from build123d import *

# Parameters (mm, degrees)
SKETCH1_R           = 5
SKETCH1_R_2         = 3
BOSS_EXTRUDE2_DEPTH = 0.5
CUT_EXTRUDE5_DEPTH  = 0.2


with BuildPart() as part:
    # Sketch1 → Boss-Extrude2 (new body)
    with BuildSketch(Plane(origin=(0, 0, 0), x_dir=(1, 0, 0), z_dir=(0, 1, 0))):
        Circle(SKETCH1_R)
        Circle(SKETCH1_R_2, mode=Mode.SUBTRACT)
    extrude(amount=BOSS_EXTRUDE2_DEPTH)

    # Sketch4 → Cut-Extrude5 (cut)
    with BuildSketch(Plane(origin=(0, 0, 0), x_dir=(1, 0, 0), z_dir=(0, 1, 0))):
        with BuildLine():
            Line((-1.227705378, 2.901045691), (-4.555523725, 1.283756278))
            ThreePointArc((-4.555523725, 1.283756278), (-4.689175287, 1.32998679), (-4.642944775, 1.463638351))
            Line((-4.642944775, 1.463638351), (-1.315126427, 3.080927764))
            ThreePointArc((-1.315126427, 3.080927764), (-1.181474866, 3.034697252), (-1.227705378, 2.901045691))
        make_face()
        with BuildLine():
            Line((0.388990404, 3.128300785), (-3.301629531, 3.391596243))
            ThreePointArc((-3.301629531, 3.391596243), (-3.394259922, 3.498458821), (-3.287397344, 3.591089212))
            Line((-3.287397344, 3.591089212), (0.403222591, 3.327793755))
            ThreePointArc((0.403222591, 3.327793755), (0.495852982, 3.220931177), (0.388990404, 3.128300785))
        make_face()
        with BuildLine():
            Line((1.902717568, 2.516761579), (-1.161805322, 4.590092101))
            ThreePointArc((-1.161805322, 4.590092101), (-1.188594305, 4.728953005), (-1.049733402, 4.755741987))
            Line((-1.049733402, 4.755741987), (2.014789488, 2.682411465))
            ThreePointArc((2.014789488, 2.682411465), (2.041578471, 2.543550562), (1.902717568, 2.516761579))
        make_face()
        with BuildLine():
            Line((2.907874144, 1.230289509), (1.290584731, 4.558107857))
            ThreePointArc((1.290584731, 4.558107857), (1.336815243, 4.691759418), (1.470466804, 4.645528907))
            Line((1.470466804, 4.645528907), (3.087756217, 1.317710559))
            ThreePointArc((3.087756217, 1.317710559), (3.041525705, 1.184058998), (2.907874144, 1.230289509))
        make_face()
        with BuildLine():
            Line((3.135129238, -0.386406272), (3.398424696, 3.304213663))
            ThreePointArc((3.398424696, 3.304213663), (3.505287274, 3.396844054), (3.597917665, 3.289981476))
            Line((3.597917665, 3.289981476), (3.334622208, -0.400638459))
            ThreePointArc((3.334622208, -0.400638459), (3.22775963, -0.49326885), (3.135129238, -0.386406272))
        make_face()
        with BuildLine():
            Line((2.523590032, -1.900133436), (4.596920554, 1.164389454))
            ThreePointArc((4.596920554, 1.164389454), (4.735781458, 1.191178437), (4.76257044, 1.052317534))
            Line((4.76257044, 1.052317534), (2.689239918, -2.012205357))
            ThreePointArc((2.689239918, -2.012205357), (2.550379015, -2.038994339), (2.523590032, -1.900133436))
        make_face()
        with BuildLine():
            Line((1.237117962, -2.905290012), (4.56493631, -1.2880006))
            ThreePointArc((4.56493631, -1.2880006), (4.698587871, -1.334231111), (4.65235736, -1.467882672))
            Line((4.65235736, -1.467882672), (1.324539012, -3.085172085))
            ThreePointArc((1.324539012, -3.085172085), (1.190887451, -3.038941573), (1.237117962, -2.905290012))
        make_face()
        with BuildLine():
            Line((-0.379577819, -3.132545106), (3.311042116, -3.395840564))
            ThreePointArc((3.311042116, -3.395840564), (3.403672507, -3.502703142), (3.296809929, -3.595333533))
            Line((3.296809929, -3.595333533), (-0.393810006, -3.332038076))
            ThreePointArc((-0.393810006, -3.332038076), (-0.486440397, -3.225175498), (-0.379577819, -3.132545106))
        make_face()
        with BuildLine():
            Line((-1.893304983, -2.521005901), (1.171217907, -4.594336423))
            ThreePointArc((1.171217907, -4.594336423), (1.19800689, -4.733197326), (1.059145987, -4.759986309))
            Line((1.059145987, -4.759986309), (-2.005376904, -2.686655787))
            ThreePointArc((-2.005376904, -2.686655787), (-2.032165886, -2.547794883), (-1.893304983, -2.521005901))
        make_face()
        with BuildLine():
            Line((-2.898461559, -1.234533831), (-1.281172147, -4.562352178))
            ThreePointArc((-1.281172147, -4.562352178), (-1.327402658, -4.69600374), (-1.461054219, -4.649773228))
            Line((-1.461054219, -4.649773228), (-3.078343632, -1.32195488))
            ThreePointArc((-3.078343632, -1.32195488), (-3.03211312, -1.188303319), (-2.898461559, -1.234533831))
        make_face()
        with BuildLine():
            Line((-3.125716653, 0.382161951), (-3.389012111, -3.308457984))
            ThreePointArc((-3.389012111, -3.308457984), (-3.495874689, -3.401088375), (-3.58850508, -3.294225797))
            Line((-3.58850508, -3.294225797), (-3.325209623, 0.396394138))
            ThreePointArc((-3.325209623, 0.396394138), (-3.218347045, 0.489024529), (-3.125716653, 0.382161951))
        make_face()
        with BuildLine():
            Line((-2.514177448, 1.895889115), (-4.58750797, -1.168633775))
            ThreePointArc((-4.58750797, -1.168633775), (-4.726368873, -1.195422758), (-4.753157856, -1.056561855))
            Line((-4.753157856, -1.056561855), (-2.679827334, 2.007961035))
            ThreePointArc((-2.679827334, 2.007961035), (-2.54096643, 2.034750018), (-2.514177448, 1.895889115))
        make_face()
    extrude(amount=CUT_EXTRUDE5_DEPTH, mode=Mode.SUBTRACT)


solid = part.part
Could you check a few things on this model? Use its own coordinates, in mm. Round coordinates to 2 decimals unless told otherwise and drop trailing zeros. Write each loop counter-clockwise with the first axis right and the second up, starting at its lowest first coordinate (ties: lowest second). Pieces come first, ordered by that corner, then holes. Notation, with made-up numbers: (87.5, -5.75) -> (91.5, -5.75) arc R15 cw to (91.5, 6.25) -> close; hole circle Ø8 at (-39, 7). An arc over 180 degrees is marked (long way). Use a Markdown table: item, result.
1. Please list where these lines run through material, in increasing order: probe 1 along X at (y, z) = (0.3, 0); probe 2 along Z at (x, y) = (0, 0.15); probe 3 along X at (y, z) = (0.15, 4).
Answer key:
| item | result |
|---|---|
| probe 1 | x = -5 to -3, 3 to 5 |
| probe 2 | z = -5 to -4.05, -3.8 to -3.36, -3.16 to -3, 3 to 3.16, 3.36 to 3.8, 4.04 to 5 |
| probe 3 | x = -3 to -1.78, -1.55 to -0.06, 0.29 to 3 |
2. If we section it at A-A (x = 0.75): List the corners of the cut face in (y, z) for me, then the cut area to 3 significant figures.
Answer key:
| item | result |
|---|---|
| outline | (0, -4.94) -> (0.5, -4.94) -> (0.5, -2.9) -> (0, -2.9) -> (0, -3.3) -> (0.2, -3.3) -> (0.2, -3.54) -> (0, -3.54) -> close; (0, 2.9) -> (0.5, 2.9) -> (0.5, 4.94) -> (0, 4.94) -> (0, 4.55) -> (0.2, 4.55) -> (0.2, 4.31) -> (0, 4.31) -> (0, 3.41) -> (0.2, 3.41) -> (0.2, 3.21) -> (0, 3.21) -> close |
| area | 1.90 mm^2 |
3. If we section it at B-B (z = 0): List the corners of the cut face in (x, y) for me, then the cut area to 3 significant figures.
Answer key:
| item | result |
|---|---|
| outline | (-5, 0) -> (-4.04, 0) -> (-4.04, 0.2) -> (-3.8, 0.2) -> (-3.8, 0) -> (-3.35, 0) -> (-3.35, 0.2) -> (-3.15, 0.2) -> (-3.15, 0) -> (-3, 0) -> (-3, 0.5) -> (-5, 0.5) -> close; (3, 0) -> (3.16, 0) -> (3.16, 0.2) -> (3.36, 0.2) -> (3.36, 0) -> (3.81, 0) -> (3.81, 0.2) -> (4.05, 0.2) -> (4.05, 0) -> (5, 0) -> (5, 0.5) -> (3, 0.5) -> close |
| area | 1.82 mm^2 |
4. If we section it at D-D (x = 4): List the corners of the cut face in (y, z) for me, then the cut area to 3 significant figures.
Answer key:
| item | result |
|---|---|
| outline | (0, -3) -> (0.5, -3) -> (0.5, 3) -> (0, 3) -> (0, 1.78) -> (0.2, 1.78) -> (0.2, 1.56) -> (0, 1.56) -> (0, 0.07) -> (0.2, 0.07) -> (0.2, -0.28) -> (0, -0.28) -> close |
| area | 2.88 mm^2 |
5. If we section it at C-C (y = 0.4): List the corners of the cut face in (x, z) for me.
Answer key:
| item | result |
|---|---|
| outline | circle Ø10 at (0, 0); hole circle Ø6 at (0, 0) |
